Input: part model. Units: mm. Frame: model coordinates. A direction names the side the tool comes from. Coordinates: 2 decimals unless noted, no trailing zeros. Order: outer loops, then holes, each group sorted by start corner. A loop starts at its lowest first (then second) coordinate and runs counter-clockwise, first axis right, second up. Notation, with made-up numbers: M 28,77.5 L 76,77.5 A30 cw 76,101.5 Z; hole C 66,-16.75 d4. An arc over 180 degrees is marked long. Answer in a Markdown table with one row per item.
from build123d import *

# Parameters (mm, degrees)
SKETCH1_R           = 5.565
BOSS_EXTRUDE1_DEPTH = 10
SKETCH2_R           = 5
BOSS_EXTRUDE2_DEPTH = 30
BOSS_EXTRUDE3_START = 40
SKETCH3_R           = 5
BOSS_EXTRUDE3_DEPTH = 40
FILLET2_R           = 5


with BuildPart() as part:
    # Sketch1 → Boss-Extrude1 (new, symmetric)
    with BuildSketch(Plane.XY):
        Circle(SKETCH1_R)
    extrude(amount=BOSS_EXTRUDE1_DEPTH, both=True)

    # Sketch2 → Boss-Extrude2 (add)
    with BuildSketch(Plane.XY.offset(10)):
        Circle(SKETCH2_R)
    extrude(amount=BOSS_EXTRUDE2_DEPTH)

    # Sketch3 → Boss-Extrude3 (add)
    with BuildSketch(Plane(origin=(0, 0, -10), x_dir=(-1, 0, 0), z_dir=(0, 0, -1)).offset(BOSS_EXTRUDE3_START)):
        with Locations(Location((0, 0, 0), (0, 0, 180))):
            Circle(SKETCH3_R)
    extrude(amount=-BOSS_EXTRUDE3_DEPTH)

    # Fillet2
    # the kernel refuses this fillet: 5 mm, written as the material it adds along each edge
    with BuildSketch(Plane(origin=(0, 0, 10), x_dir=(1, 0, 0), z_dir=(0, -1, 0))) as fillet2_piece_1:
        with BuildLine():
            CenterArc((10, 2.308847115), FILLET2_R, 180, 27.501344198)
            Line((5, 2.308847115), (4.9, 2.308847115))
            Line((4.9, 2.308847115), (4.9, 0))
            Line((4.9, 0), (5, -0.1))
            ThreePointArc((5, -0.1), (5.2825, -0.1), (5.4763, -0.046176942))
            Line((5.4763, -0.046176942), (5.565, 0))
        make_face()
    revolve(axis=Axis((0, 0, 10), (0, 0, 1)))
    with BuildSketch(Plane(origin=(0, 0, -10), x_dir=(1, 0, 0), z_dir=(0, 1, 0))) as fillet2_piece_2:
        with BuildLine():
            CenterArc((10, 2.308847115), FILLET2_R, 180, 27.501344198)
            Line((5, 2.308847115), (4.9, 2.308847115))
            Line((4.9, 2.308847115), (4.9, 0))
            Line((4.9, 0), (5, -0.1))
            ThreePointArc((5, -0.1), (5.2825, -0.1), (5.4763, -0.046176942))
            Line((5.4763, -0.046176942), (5.565, 0))
        make_face()
    revolve(axis=Axis((0, 0, -10), (0, 0, -1)))


solid = part.part
1) Contact query for flat-ended pins moving along their axis: pin 1 (2 mm diameter, centred on x = 3, z = 20, fed in from +Y); pin 2 (3 mm diameter, centred on x = 2.5, z = 10, fed in from +Y); pin 3 (1 mm diameter, centred on x = -1, z = -34.5, fed in from -Y). Output: stop coordinate, or through.
Resolved:
| item | result |
|---|---|
| pin 1 | stops at y = 4.58 |
| pin 2 | stops at y = 5.47 |
| pin 3 | stops at y = -4.97 |
2) Material intervals for probe 1 along Y at (x, z) = (0, -39); probe 2 along Y at (x, z) = (3.5, -27.5); probe 3 along X at (y, z) = (-2.5, 25), sorted ascending.
Resolved:
| item | result |
|---|---|
| probe 1 | y = -5 to 5 |
| probe 2 | y = -3.57 to 3.57 |
| probe 3 | x = -4.33 to 4.33 |
3) Cut plane A-A, the plane y = 0. Output: boundary loops of the cut face in (x, z) (3 decimals), and give its area (3 significant figures).
Resolved:
| item | result |
|---|---|
| outline | M -5.565,-10 A5 cw -5,-12.309 L -5,-50 L 5,-50 L 5,-12.309 A5 cw 5.565,-10 L 5.565,10 A5 cw 5,12.309 L 5,40 L -5,40 L -5,12.309 A5 cw -5.565,10 Z |
| area | 924 mm2 |
4) Reachability of faces 1 (the face through (-1.08, -4.88, 25.96)), 2 (the face through (-5, 0, -31)), 3 (the face through (0, 0, 40)) from +Z, -Z, +X, -X, +Y, -Y: full face, straight path, thin tool, end or side. Return the list, or none.
Resolved:
| item | result |
|---|---|
| face 1 | +Z |
| face 2 | -Z |
| face 3 | +Z, +X, -X, +Y, -Y |
5) Cut plane D-D, the plane z = 30.5. Output: boundary loops of the cut face in (x, y).
Resolved:
| item | result |
|---|---|
| outline | C 0,0 d10 |
6) Cut plane C-C, the plane z = -5.5. Output: boundary loops of the cut face in (x, y) (3 decimals).
Resolved:
| item | result |
|---|---|
| outline | C 0,0 d11.13 |
